from build123d import *

# Parameters (mm, degrees)
SKETCH_1_W                  = 56.1
SKETCH_1_H                  = 20
EXTRUDE_1_DEPTH             = 5
EXTRUDE_2_DEPTH             = 30
HOLE_WIZARD_M41_D           = 4.5
HOLE_WIZARD_M41_CSINK_D     = 8.96
HOLE_WIZARD_M41_CSINK_ANGLE = 90
FILLET_1_R                  = 2


with BuildPart() as part:
    # Эскиз1 → Бобышка-Вытянуть1 (new body)
    with BuildSketch(Plane.XY):
        with Locations((28.05, 10)):
            Rectangle(SKETCH_1_W, SKETCH_1_H)
    extrude(amount=EXTRUDE_1_DEPTH)

    # Эскиз2 → Бобышка-Вытянуть2 (add)
    with BuildSketch(Plane.XY.offset(5)):
        with BuildLine():
            Line((19.05, 12.02562419), (19.05, 20))
            Line((19.05, 20), (0, 20))
            Line((0, 20), (0, 0))
            Line((0, 0), (13.05, 0))
            Line((13.05, 0), (13.652765995, 0.502304996))
            ThreePointArc((13.652765995, 0.502304996), (17.633841318, 5.663293246), (19.05, 12.02562419))
        make_face()
        with BuildLine():
            Line((56.1, 20), (37.05, 20))
            Line((37.05, 20), (37.05, 12.02562419))
            ThreePointArc((37.05, 12.02562419), (38.466158682, 5.663293246), (42.447234005, 0.502304996))
            Line((42.447234005, 0.502304996), (43.05, 0))
            Line((43.05, 0), (56.1, 0))
            Line((56.1, 0), (56.1, 20))
        make_face()
    extrude(amount=EXTRUDE_2_DEPTH)

    # Зенковка для  винта с потайной головкой с внутренним шестигранником M41 (through all)
    with Locations(Plane(origin=(9.525, 10, 35), x_dir=(1, 0, 0), z_dir=(0, 0, 1))):
        with Locations((0, 0), (37.05, 0)):
            CounterSinkHole(HOLE_WIZARD_M41_D / 2, HOLE_WIZARD_M41_CSINK_D / 2, counter_sink_angle=HOLE_WIZARD_M41_CSINK_ANGLE)

    # Скругление1
    fillet_1_edges = [part.edges().sort_by_distance(p)[0] for p in [
        (28.05, 0, 5),
    ]]
    fillet(fillet_1_edges, radius=FILLET_1_R)
    fillet_1_2_edges = [part.edges().sort_by_distance(p)[0] for p in [
        (13.05, 0, 19),
    ]]
    fillet(fillet_1_2_edges, radius=FILLET_1_R)
    fillet_1_3_edges = [part.edges().sort_by_distance(p)[0] for p in [
        (43.05, 0, 19.000000047),
    ]]
    fillet(fillet_1_3_edges, radius=FILLET_1_R)


solid = part.part
Geometry: final body of the model. Coordinates: model frame, mm. A direction names the side the tool comes from. Coordinates: 2 decimals unless noted, no trailing zeros. Order: outer loops, then holes, each group sorted by start corner. A loop starts at its lowest first (then second) coordinate and runs counter-clockwise, first axis right, second up.
1) Section B-B (z = 2). Return loops of the section in (x, y) (3 decimals).
Result sheet:
outline: (0, 0) - (56.1, 0) - (56.1, 20) - (0, 20) - close; hole circle Ø4.5 at (9.525, 10); hole circle Ø4.5 at (46.575, 10)
2) Section D-D (x = 21.5). Return loops of the section in (y, z).
Result sheet:
outline: (0, 0) - (20, 0) - (20, 5) - (2, 5) arc R2 ccw to (0, 3) - close
3) Set-up query: faces 1 (the flat face through (19.05, 16, 20)), 2 (the cylindrical face through (28.27, 0.57, 4.4)), 3 (the flat face through (28, 0, 2)). Return all of +Z, -Z, +X, -X, +Y, -Y with unobstructed straight access to the full face (end or side cutting, diameter ignored); none if empty.
Result sheet:
face 1: +Z, +Y, -Y
face 2: +Z, -Y
face 3: +Z, -Z, +X, -X, -Y
4) Ray query, probe 1 along X at (y, z) = (14.25, 23); probe 2 along X at (y, z) = (10, 21.5) (3 decimals); probe 3 along X at (y, z) = (11.75, 25.5). Return the intervals inside material, ascending.
Result sheet:
probe 1: x = 0 to 19.05, 37.05 to 56.1
probe 2: x = 0 to 7.275, 11.775 to 18.913, 37.187 to 44.325, 48.825 to 56.1
probe 3: x = 0 to 8.11, 10.94 to 19.05, 37.05 to 45.16, 47.99 to 56.1
5) First-contact query: P1, Ø6, axis at x = 9.525, y = 10, coming from the +Z side; P2, Ø5.5, axis at x = 28.5, y = 11, coming from the +Z side. Flat tips, straight axial feed; report the tip coordinate or a pass-through.
Result sheet:
P1: stops at z = 33.52
P2: stops at z = 5
6) Draft query along X for faces 4 (the flat face through (9, 15, 35)), 5 (the flat face through (0, 10, 17)), 6 (the cylindrical face through (8.32, 11.9, 16.16)). Return one class per face: released by +X, released by -X, zero draft, split by the parting line, or undercut.
Result sheet:
face 4: zero draft
face 5: released by -X
face 6: undercut
7) Section C-C (y = 10). Return loops of the section in (x, z) (3 decimals), then the cut area to 3 significant figures.
Result sheet:
outline: (0, 0) - (7.275, 0) - (7.275, 32.77) - (5.045, 35) - (0, 35) - close; (11.775, 0) - (44.325, 0) - (44.325, 32.77) - (42.095, 35) - (37.187, 35) - (37.187, 5) - (18.913, 5) - (18.913, 35) - (14.005, 35) - (11.775, 32.77) - close; (48.825, 0) - (56.1, 0) - (56.1, 35) - (51.055, 35) - (48.825, 32.77) - close
area: 1,090 mm2
8) Section A-A (z = 11). Return loops of the section in (x, y) (3 decimals).
Result sheet:
outline: (0, 0) - (12.326, 0) arc R2 ccw to (13.606, 0.464) - (13.653, 0.502) arc R15 ccw to (19.05, 12.026) - (19.05, 20) - (0, 20) - close; (37.05, 12.026) arc R15 ccw to (42.447, 0.502) - (42.494, 0.464) arc R2 ccw to (43.774, 0) - (56.1, 0) - (56.1, 20) - (37.05, 20) - close; hole circle Ø4.5 at (9.525, 10); hole circle Ø4.5 at (46.575, 10)
